from build123d import *

# Parameters (mm, degrees)
SZKIC1_W                    = 60
SZKIC1_H                    = 8
DODANIE_WYCI_GNI_CIE1_DEPTH = 3
ZAOKR_GLENIE1_R             = 4
SZKIC2_R                    = 1.5
WYTNIJ_WYCI_GNI_CIE1_DEPTH  = 3
SZKIC3_W                    = 2
SZKIC3_H                    = 6
DODANIE_WYCI_GNI_CIE2_DEPTH = 4
WYTNIJ_WYCI_GNI_CIE2_REACH  = 52.14
SZKIC4_R                    = 1
ZAOKR_GLENIE2_R             = 2


with BuildPart() as part:
    # Szkic1 → Dodanie-wyciągnięcie1 (new body)
    with BuildSketch(Plane.XY):
        with Locations((30, 4)):
            Rectangle(SZKIC1_W, SZKIC1_H)
    extrude(amount=DODANIE_WYCI_GNI_CIE1_DEPTH)

    # Zaokrąglenie1
    zaokr_glenie1_edges = [part.edges().sort_by_distance(p)[0] for p in [
        (0, 0, 1.5),
        (0, 8, 1.5),
        (60, 8, 1.5),
        (60, 0, 1.5),
    ]]
    fillet(zaokr_glenie1_edges, radius=ZAOKR_GLENIE1_R - 0.0001)  # a hair under: the kernel refuses the full size

    # Szkic2 → Wytnij-wyciągnięcie1 (cut)
    with BuildSketch(Plane.XY.offset(3)):
        with Locations((4, 4)):
            Circle(SZKIC2_R)
        with Locations((56, 4)):
            Circle(SZKIC2_R)
    extrude(amount=-WYTNIJ_WYCI_GNI_CIE1_DEPTH, mode=Mode.SUBTRACT)

    # Szkic3 → Dodanie-wyciągnięcie2 (add)
    with BuildSketch(Plane.XY.offset(3)):
        with Locations((12, 3)):
            Rectangle(SZKIC3_W, SZKIC3_H)
    extrude(amount=DODANIE_WYCI_GNI_CIE2_DEPTH)

    # Szkic4 → Wytnij-wyciągnięcie2 (cut, up to next)
    with BuildSketch(Plane.ZY.offset(-11), mode=Mode.PRIVATE) as wytnij_wyci_gni_cie2_sk1:
        with Locations((5, 3)):
            Circle(SZKIC4_R)
    wytnij_wyci_gni_cie2_tool1 = extrude(wytnij_wyci_gni_cie2_sk1.sketch, amount=-WYTNIJ_WYCI_GNI_CIE2_REACH, mode=Mode.PRIVATE) & part.part
    add(wytnij_wyci_gni_cie2_tool1.solids().sort_by_distance((11, 3, 5))[0], mode=Mode.SUBTRACT)

    # Zaokrąglenie2
    zaokr_glenie2_edges = [part.edges().sort_by_distance(p)[0] for p in [
        (12, 0, 7),
        (12, 6, 7),
    ]]
    fillet(zaokr_glenie2_edges, radius=ZAOKR_GLENIE2_R)


solid = part.part
CAD build for the part. Positions are in the model's coordinates, mm. A direction names the side the tool comes from. Round coordinates to 2 decimals unless told otherwise and drop trailing zeros. Loops run counter-clockwise (first coordinate to the right, second up) from the corner with the lowest first, then second, coordinate; pieces in that order, holes last. Notation, with made-up numbers: (-19, 2.25) - (19, 2.25) arc R10 cw to (19, 13.25) - close; hole circle Ø5 at (70, 11.25). An arc over 180 degrees is marked (long way). Put each result on its own line as item: value.
1. Slice it at A-A on z = 2.25. Give the number of separate pieces and of enclosed holes in the cut face, and give its area (3 significant figures).
Geometry check:
separate pieces: 1
enclosed holes: 2
area: 452 mm²
2. Slice it at B-B on x = 55.5. List the corners of the cut face in (y, z).
Geometry check:
outline: (0, 0) - (2.59, 0) - (2.59, 3) - (0, 3) - close; (5.41, 0) - (8, 0) - (8, 3) - (5.41, 3) - close
3. 3-axis set-ups, long thin cutter, end or side, ignore diameter. For faces 1 (the flat face through (11, 4, 4)), 2 (the flat face through (30, 0, 1)), 3 (the flat face through (12, 6, 4)): which of +Z, -Z, +X, -X, +Y, -Y reach the whole face in a straight line?
Geometry check:
face 1: +Z, -X, +Y, -Y
face 2: +Z, -Z, +X, -X, -Y
face 3: +Z, +X, -X, +Y
4. Two-plate mould, pull along X, no slides. Class faces 4 (the flat face through (13, 4, 4)), 5 (the flat face through (12, 3, 7)), 6 (the cylindrical face through (57.43, 4.45, 1.52)), 7 (the cylindrical face through (5.43, 4.45, 1.52)): released by +X, released by -X, zero draft, split by the parting line, or undercut.
Geometry check:
face 4: released by +X
face 5: zero draft
face 6: undercut
face 7: undercut
5. Wall check: line 1 (Y direction, x = 56, z = 1.5); line 2 (X direction, y = 4.5, z = 0.75); line 3 (X direction, y = 5.25, z = 1). Give the ranges that are in metal, low to high.
Geometry check:
line 1: 0 to 2.5, 5.5 to 8
line 2: 0.03 to 2.59, 5.41 to 54.59, 57.41 to 59.97
line 3: 0.2 to 3.17, 4.83 to 55.17, 56.83 to 59.8
6. Pin check, flat tips, straight feed: P1, Ø4, axis at x = 29, y = 3.5, coming from the +Z side; P2, Ø1.6, axis at x = 11.5, z = 4, coming from the +Y side; P3, Ø1, axis at y = 5, z = 5, coming from the +X side. Stop position of each tip, or through.
Geometry check:
P1: z = 3
P2: y = 6
P3: x = 13
7. Slice it at C-C on z = 5.5. List the corners of the cut face in (x, y), and give its area (3 significant figures).
Geometry check:
outline: (11, 0.06) - (13, 0.06) - (13, 2.13) - (11, 2.13) - close; (11, 3.87) - (13, 3.87) - (13, 5.94) - (11, 5.94) - close
area: 8.28 mm²
8. Slice it at D-D on y = 1.5. List the corners of the cut face in (x, z), and give its area (3 significant figures).
Geometry check:
outline: (0.88, 0) - (59.12, 0) - (59.12, 3) - (13, 3) - (13, 6.94) - (11, 6.94) - (11, 3) - (0.88, 3) - close
area: 183 mm²
